Can you work these out from the model? Positions are in its coordinate system, mm. A direction names the side the tool comes from. Round coordinates to 2 decimals unless told otherwise and drop trailing zeros. Order: outer loops, then holes, each group sorted by start corner. A loop starts at its lowest first (then second) coordinate and runs counter-clockwise, first axis right, second up.
Q1. If I drill on line 1 (Y direction, x = 0, z = -2.25); line 2 (Z direction, x = 4.75, y = -0.75); line 3 (Z direction, x = 0, y = -0.75), over which ranges is the centre line in solid material (lowest first)?
Q2. If we section it at B-B (y = 5): Please give me the cut outline in (x, z), plus the area to 3 significant figures.
Q3. For faces 1 (the face through (-0.867, -3.905, -10.549)), 2 (the face through (-4, -2, 0)), 3 (the face through (-6, 0, -6)), which set-ups out of +Z, -Z, +X, -X, +Y, -Y let a thin tool reach every point of the face, with its end or its side?
Q4. We'd pull the mould along Y, two halves only. Please class faces 4 (the face through (-1.19, -5.37, 0.99)), 5 (the face through (-0.596, -2.685, -2.93)), 6 (the face through (-1.42, -3.92, -5)), 7 (the face through (0, 0, -8)): pulls with the +Y half, pulls with the -Y half, needs draft (parallel to the pull), parting line crosses it, or undercut.
Q5. Will these pins go through, and if not, where does the flat tip stop? P1, Ø6, axis at x = -1.5, z = -10.5, coming from the +Y side; P2, Ø1.5, axis at y = 0, z = -10, coming from the +X side; P3, Ø1.6, axis at x = 0.5, y = -0.5, coming from the +Z side; P4, Ø7, axis at x = 0, y = 0, coming from the +Z side.
Q6. If we section it at C-C (z = -1.75): Please give me the cut outline in (x, y).
Q7. If we section it at A-A (x = 0): Please give me the cut outline in (y, z).
from build123d import *

# Parameters (mm, degrees)
SKETCH1_R    = 5.5
FLANGE_DEPTH = 2
BARREL_START = -14
SKETCH2_R    = 4
BARREL_DEPTH = 14
NUT_START    = -7
SKETCH3_R    = 6
NUT_DEPTH    = 2
SOCKET_START = 2
SKETCH4_R    = 2.75
SOCKET_DEPTH = 10


with BuildPart() as part:
    # Sketch1 → Flange (new body)
    with BuildSketch(Plane.XY):
        Circle(SKETCH1_R)
    extrude(amount=FLANGE_DEPTH)

    # Sketch2 → Barrel (add)
    with BuildSketch(Plane.XY.offset(BARREL_START)):
        Circle(SKETCH2_R)
    extrude(amount=BARREL_DEPTH)

    # Sketch3 → Nut (add)
    with BuildSketch(Plane.XY.offset(NUT_START)):
        Circle(SKETCH3_R)
    extrude(amount=NUT_DEPTH)

    # Sketch4 → Socket (cut)
    with BuildSketch(Plane.XY.offset(SOCKET_START)):
        Circle(SKETCH4_R)
    extrude(amount=-SOCKET_DEPTH, mode=Mode.SUBTRACT)


solid = part.part
Solution:
1. line 1: y = -4 to -2.75, 2.75 to 4
1. line 2: z = -7 to -5, 0 to 2
1. line 3: z = -14 to -8
2. outline: (-3.32, -7) - (3.32, -7) - (3.32, -5) - (-3.32, -5) - close; (-2.29, 0) - (2.29, 0) - (2.29, 2) - (-2.29, 2) - close
2. area: 22.4 mm2
3. face 1: -Z
3. face 2: none
3. face 3: +Z, -Z
4. face 4: parting line crosses it
4. face 5: undercut
4. face 6: needs draft
4. face 7: undercut
5. P1: stops at y = 4
5. P2: stops at x = 4
5. P3: stops at z = -8
5. P4: stops at z = 2
6. outline: circle Ø8 at (0, 0); hole circle Ø5.5 at (0, 0)
7. outline: (-6, -7) - (-4, -7) - (-4, -14) - (4, -14) - (4, -7) - (6, -7) - (6, -5) - (4, -5) - (4, 0) - (5.5, 0) - (5.5, 2) - (2.75, 2) - (2.75, -8) - (-2.75, -8) - (-2.75, 2) - (-5.5, 2) - (-5.5, 0) - (-4, 0) - (-4, -5) - (-6, -5) - close
